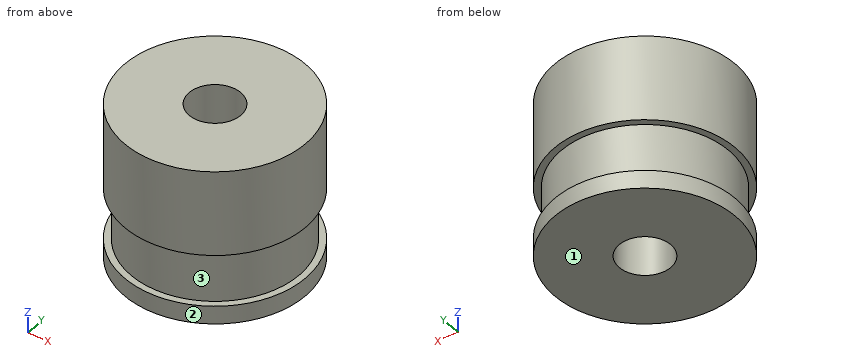
```python
from build123d import *

# Parameters (mm, degrees)
ESQUISSE1_R        = 35
ESQUISSE1_R_2      = 10
BOSS_EXTRU_1_DEPTH = 7
ESQUISSE2_R        = 32.5
ESQUISSE2_R_2      = 10
BOSS_EXTRU_2_DEPTH = 20
ESQUISSE3_R        = 35
ESQUISSE3_R_2      = 10
BOSS_EXTRU_3_DEPTH = 33


with BuildPart() as part:
    # Esquisse1 → Boss.-Extru.1 (new body)
    with BuildSketch(Plane.XY):
        Circle(ESQUISSE1_R)
        Circle(ESQUISSE1_R_2, mode=Mode.SUBTRACT)
    extrude(amount=BOSS_EXTRU_1_DEPTH)

    # Esquisse2 → Boss.-Extru.2 (add)
    with BuildSketch(Plane.XY.offset(7)):
        Circle(ESQUISSE2_R)
        Circle(ESQUISSE2_R_2, mode=Mode.SUBTRACT)
    extrude(amount=BOSS_EXTRU_2_DEPTH)

    # Esquisse3 → Boss.-Extru.3 (add)
    with BuildSketch(Plane.XY.offset(27)):
        Circle(ESQUISSE3_R)
        Circle(ESQUISSE3_R_2, mode=Mode.SUBTRACT)
    extrude(amount=BOSS_EXTRU_3_DEPTH)


solid = part.part
```
Work out the finished part from the listing and answer in its coordinate system (mm). Face numbers are marked on the shaded views. Give positions to 0.01 mm unless a question says otherwise; leave off trailing zeros. Loops run counter-clockwise (first coordinate to the right, second up) from the corner with the lowest first, then second, coordinate; pieces in that order, holes last. Notation, with made-up numbers: (35, -32.75) - (77, -32.75) arc R18 cw to (77, -0.75) - close; hole circle Ø11 at (-15, 68.25). An arc over 180 degrees is marked (long way). One line per question, with ' | ' between items.
(1) Straight lines are drawn through the part: probe 1 along Y at (x, z) = (0, 26); probe 2 along X at (y, z) = (2, 13); probe 3 along Z at (x, y) = (-5.5, 32.5). For each, find the intervals that lie inside material, in ascending order.
Recorded:
probe 1: y = -32.5 to -10, 10 to 32.5 | probe 2: x = -32.44 to -9.8, 9.8 to 32.44 | probe 3: z = 0 to 7, 27 to 60
(2) The mould has two halves that part along Z. Classify the marked faces 1, 2 and 3: +Z half, -Z half, draft (parallel to the pull), parting line (faces both ways), or undercut.
Recorded:
face 1: -Z half | face 2: draft | face 3: undercut
(3) The part is cut by section D-D (x = -16). Write down the section's boundary in (y, z).
Recorded:
outline: (-31.13, 0) - (31.13, 0) - (31.13, 7) - (28.29, 7) - (28.29, 27) - (31.13, 27) - (31.13, 60) - (-31.13, 60) - (-31.13, 27) - (-28.29, 27) - (-28.29, 7) - (-31.13, 7) - close
(4) The part is cut by section C-C (z = 43.5). Write down the section's boundary in (x, y), then the cut area to 3 significant figures.
Recorded:
outline: circle Ø70 at (0, 0); hole circle Ø20 at (0, 0) | area: 3,530 mm²
(5) The part is cut by section A-A (y = 0). Write down the section's boundary in (x, z).
Recorded:
outline: (-35, 0) - (-10, 0) - (-10, 60) - (-35, 60) - (-35, 27) - (-32.5, 27) - (-32.5, 7) - (-35, 7) - close; (10, 0) - (35, 0) - (35, 7) - (32.5, 7) - (32.5, 27) - (35, 27) - (35, 60) - (10, 60) - close
(6) Each of these flat-tipped pins is pushed along its axis until it touches: pin 1 Ø1.5 at (x, y) = (26, -2) entering from -Z; pin 2 Ø8 at (x, z) = (17, 21.5) entering from +Y; pin 3 Ø6 at (x, z) = (17, 50.5) entering from +Y; pin 4 Ø3 at (x, z) = (20.5, 38) entering from +Y. Where does it stop, or does it pass through?
Recorded:
pin 1: stops at z = 0 | pin 2: stops at y = 29.79 | pin 3: stops at y = 32.08 | pin 4: stops at y = 29.39
